Build history of the part. All positions in model axes, mm. A direction names the side the tool comes from. Round coordinates to 2 decimals unless told otherwise and drop trailing zeros. Order: outer loops, then holes, each group sorted by start corner. A loop starts at its lowest first (then second) coordinate and runs counter-clockwise, first axis right, second up. Notation, with made-up numbers: M 65,-21.5 L 76,-21.5 A25 ccw 76,-5.5 Z; hole C -23,41.25 d3. An arc over 180 degrees is marked long. One line per item, written item: value. Start each with the question number.
Item 1: Band-saw the part on A-A, the plane y = 29.94. Write the cut outline in (x, z), then the cut area to 3 significant figures.
Item 2: Band-saw the part on B-B, the plane x = 2.75. Write the cut outline in (y, z).
Item 3: Band-saw the part on D-D, the plane y = 21. Write the cut outline in (x, z), then the cut area to 3 significant figures.
Item 4: Probe L1, parallel to X at y = 60.7, z = 1.2; L2, parallel to X at y = 35.2, z = 1.5; L3, parallel to Y at x = 10.25, z = 0.95. List the from-to ranges inside material, lowest first.
Item 5: Two-plate mould, pull along Y, no slides. Class faces 1 (the cylindrical face through (0.57, 44.1, 0.99)), 2 (the flat face through (0, 32, 1)), 3 (the cylindrical face through (3.2, 42.8, 1)), 4 (the flat face through (8, 67.93, 1)): +Y half, -Y half, draft (parallel to the pull), parting line (faces both ways), or undercut.
Item 6: Tool access for faces 5 (the flat face through (16.2, 33, 1)), 6 (the flat face through (10.2, 49, 1)), 7 (the flat face through (3, 52.7, 1)), 8 (the cylindrical face through (15.63, 53.3, 0.99)): list every direction of +Z, -Z, +X, -X, +Y, -Y with a clear straight run to the whole face (end or side of a thin tool).
Item 7: Pin check, flat tips, straight feed: pin 1 (0.6 mm diameter, centred on y = 47.5, z = 1, fed in from -X); pin 2 (0.6 mm diameter, centred on x = 13, z = 1, fed in from -Y). Stop position of each tip, or through.
Item 8: Band-saw the part on C-C, the plane z = 0.5. Give the number of separate pieces and of enclosed holes in the cut face, then the cut area to 3 significant figures.
```python
from build123d import *

# Parameters (mm, degrees)
SKETCH1_R           = 0.75
SKETCH1_R_2         = 0.95
SKETCH1_W           = 4.2
SKETCH1_H           = 8
BOSS_EXTRUDE1_DEPTH = 2


with BuildPart() as part:
    # Sketch1 → Boss-Extrude1 (new body)
    with BuildSketch(Plane.XY):
        with BuildLine():
            Line((4, 44.7), (4, 52.7))
            Line((4, 52.7), (2, 52.7))
            ThreePointArc((2, 52.7), (0.585786438, 53.285786438), (0, 54.7))
            Line((0, 54.7), (0, 67.93))
            Line((0, 67.93), (16.2, 67.93))
            Line((16.2, 67.93), (16.2, 54.7))
            ThreePointArc((16.2, 54.7), (15.614213562, 53.285786438), (14.2, 52.7))
            Line((14.2, 52.7), (12.2, 52.7))
            Line((12.2, 52.7), (12.2, 44.7))
            Line((12.2, 44.7), (14.2, 44.7))
            ThreePointArc((14.2, 44.7), (15.614213562, 44.114213562), (16.2, 42.7))
            Line((16.2, 42.7), (16.2, 22.44))
            ThreePointArc((16.2, 22.44), (15.614213562, 21.025786438), (14.2, 20.44))
            Line((14.2, 20.44), (12.2, 20.44))
            Line((12.2, 20.44), (12.2, 12.44))
            Line((12.2, 12.44), (10.2, 12.44))
            Line((10.2, 12.44), (10.2, 20.44))
            Line((10.2, 20.44), (6, 20.44))
            Line((6, 20.44), (6, 12.44))
            Line((6, 12.44), (4, 12.44))
            Line((4, 12.44), (4, 20.44))
            Line((4, 20.44), (2, 20.44))
            ThreePointArc((2, 20.44), (0.585786438, 21.025786438), (0, 22.44))
            Line((0, 22.44), (0, 42.7))
            ThreePointArc((0, 42.7), (0.585786438, 44.114213562), (2, 44.7))
            Line((2, 44.7), (4, 44.7))
        make_face()
        with Locations((2.75, 60.7)):
            Circle(SKETCH1_R, mode=Mode.SUBTRACT)
        with Locations((13.45, 54.7)):
            Circle(SKETCH1_R, mode=Mode.SUBTRACT)
        with Locations((13.45, 42.2)):
            Circle(SKETCH1_R, mode=Mode.SUBTRACT)
        with Locations((13.45, 22.94)):
            Circle(SKETCH1_R_2, mode=Mode.SUBTRACT)
        with Locations((10.2, 29.94)):
            Circle(SKETCH1_R_2, mode=Mode.SUBTRACT)
        with Locations((6, 35.2)):
            Circle(SKETCH1_R, mode=Mode.SUBTRACT)
        with Locations((13.45, 60.7)):
            Circle(SKETCH1_R, mode=Mode.SUBTRACT)
        with Locations((10.2, 35.2)):
            Circle(SKETCH1_R, mode=Mode.SUBTRACT)
        with Locations((6, 29.94)):
            Circle(SKETCH1_R_2, mode=Mode.SUBTRACT)
        with Locations((2.75, 22.94)):
            Circle(SKETCH1_R_2, mode=Mode.SUBTRACT)
        with Locations((2.75, 42.2)):
            Circle(SKETCH1_R, mode=Mode.SUBTRACT)
        with Locations((2.75, 54.7)):
            Circle(SKETCH1_R, mode=Mode.SUBTRACT)
        with Locations((8.1, 48.7)):
            Rectangle(SKETCH1_W, SKETCH1_H, mode=Mode.SUBTRACT)
    extrude(amount=BOSS_EXTRUDE1_DEPTH)


solid = part.part
```
Output:
1. outline: M 0,0 L 5.05,0 L 5.05,2 L 0,2 Z; M 6.95,0 L 9.25,0 L 9.25,2 L 6.95,2 Z; M 11.15,0 L 16.2,0 L 16.2,2 L 11.15,2 Z
1. area: 24.8 mm²
2. outline: M 20.44,0 L 21.99,0 L 21.99,2 L 20.44,2 Z; M 23.89,0 L 41.45,0 L 41.45,2 L 23.89,2 Z; M 42.95,0 L 44.7,0 L 44.7,2 L 42.95,2 Z; M 52.7,0 L 53.95,0 L 53.95,2 L 52.7,2 Z; M 55.45,0 L 59.95,0 L 59.95,2 L 55.45,2 Z; M 61.45,0 L 67.93,0 L 67.93,2 L 61.45,2 Z
3. outline: M 0.61,0 L 15.59,0 L 15.59,2 L 0.61,2 Z
3. area: 30.0 mm²
4. L1: x = 0 to 2, 3.5 to 12.7, 14.2 to 16.2
4. L2: x = 0 to 5.25, 6.75 to 9.45, 10.95 to 16.2
4. L3: y = 12.44 to 28.99, 30.89 to 34.45, 35.95 to 67.93
5. face 1: undercut
5. face 2: draft
5. face 3: undercut
5. face 4: +Y half
6. face 5: +Z, -Z, +X, +Y, -Y
6. face 6: +Z, -Z
6. face 7: +Z, -Z, -X
6. face 8: +Z, -Z, +X
7. pin 1: stops at x = 4
7. pin 2: stops at y = 20.44
8. separate pieces: 1
8. enclosed holes: 13
8. area: 673 mm²
